Verification items for this drawing (mm, ordinates from the low corner). A direction names the side the tool comes from. Give positions to 0.01 mm unless a question says otherwise; leave off trailing zeros. Order: outer loops, then holes, each group sorted by start corner. A loop starts at its lowest first (then second) coordinate and runs counter-clockwise, first axis right, second up.
(1) Sectioned sample at A-A on y = 41. Record the cut outline in (x, z).
(2) Gauge pin test, flat ends, axial feed: pin 1 (5 mm diameter, centred on x = 64.5, z = 11.5, fed in from +Y); pin 2 (3 mm diameter, centred on x = 32, y = 2.5, fed in from -Z). Record the tip position at first contact, or that the pin passes through.
(3) Sectioned sample at D-D on z = 11.5. Record the cut outline in (x, y).
(4) Access from +Z, -Z, +X, -X, +Y, -Y to the whole of each face (thin tool, end or side, straight path). Record for the marked faces 1, 2 and 3.
(5) Scan lines: L1, parallel to X at y = 45, z = 4; L2, parallel to Y at x = 96.25, z = 7.75; L3, parallel to Y at x = 33.5, z = 1. Record each from-to range of solid material in increasing order.
(6) Sectioned sample at C-C on x = 96.25. Record the cut outline in (y, z), plus the area to 3 significant figures.
(7) Sectioned sample at B-B on z = 4.75. Record the cut outline in (x, y), plus the area to 3 significant figures.
(8) Mould release check, pull along X, two halves, no side actions. Record for the marked faces 4, 5 and 6: pulls with the +X half, pulls with the -X half, needs draft (parallel to the pull), parting line crosses it, or undercut.
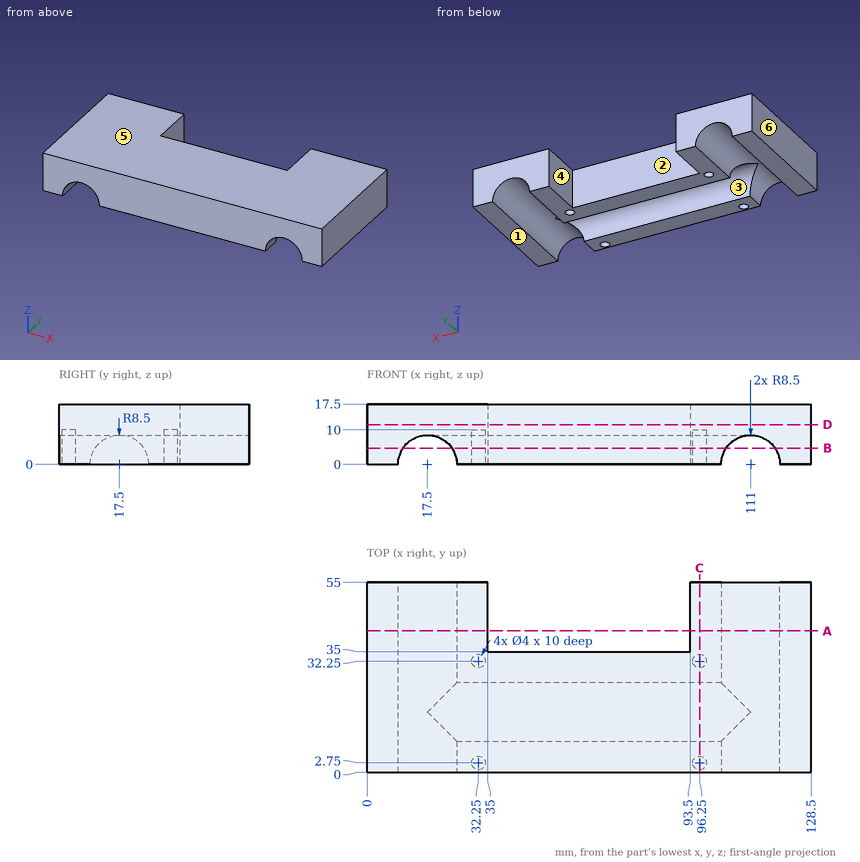
Ans:
1. outline: (0, 0) - (9, 0) arc R8.5 cw to (26, 0) - (35, 0) - (35, 17.5) - (0, 17.5) - close; (93.5, 0) - (102.5, 0) arc R8.5 cw to (119.5, 0) - (128.5, 0) - (128.5, 17.5) - (93.5, 17.5) - close
2. pin 1: stops at y = 35
2. pin 2: stops at z = 10
3. outline: (0, 0) - (128.5, 0) - (128.5, 55) - (93.5, 55) - (93.5, 35) - (35, 35) - (35, 55) - (0, 55) - close
4. face 1: -Z, +X, -X, +Y, -Y
4. face 2: +Z, -Z, +Y
4. face 3: -Z
5. L1: x = 0 to 10, 25 to 35, 93.5 to 103.5, 118.5 to 128.5
5. L2: y = 0 to 0.75, 4.75 to 14.01, 20.99 to 30.25, 34.25 to 55
5. L3: y = 0 to 1.19, 4.31 to 9.06, 25.94 to 30.69, 33.81 to 55
6. outline: (0, 0) - (0.75, 0) - (0.75, 10) - (4.75, 10) - (4.75, 0) - (9, 0) arc R8.5 cw to (26, 0) - (30.25, 0) - (30.25, 10) - (34.25, 10) - (34.25, 0) - (55, 0) - (55, 17.5) - (0, 17.5) - close
6. area: 769 mm2
7. outline: (0, 0) - (10.45, 0) - (10.45, 55) - (0, 55) - close; (24.55, 0) - (103.95, 0) - (103.95, 10.45) - (24.55, 10.45) - close; (24.55, 24.55) - (103.95, 24.55) - (103.95, 55) - (93.5, 55) - (93.5, 35) - (35, 35) - (35, 55) - (24.55, 55) - close; (118.05, 0) - (128.5, 0) - (128.5, 55) - (118.05, 55) - close; hole circle Ø4 at (32.25, 2.75); hole circle Ø4 at (32.25, 32.25); hole circle Ø4 at (96.25, 2.75); hole circle Ø4 at (96.25, 32.25)
7. area: 3,180 mm2
8. face 4: undercut
8. face 5: needs draft
8. face 6: pulls with the -X half
